from build123d import *

# Parameters (mm, degrees)
F2_SIZE = 1
F3_R    = 1


with BuildPart() as f1:
    # F0 (on Front) → F1 (revolve)
    with BuildSketch(Plane.XZ):
        Polygon((0, 4), (0, 0), (25, 0), (25, 4), (19.505045, 6), (14, 6), (14, 4), align=None)
    revolve(axis=Axis((10.323764, 0, 0), (1, 0, 0)))

    # F2
    f2_edges = [f1.edges().sort_by_distance(p)[0] for p in [
        (0, 0, -4),
    ]]
    chamfer(f2_edges, length=F2_SIZE)

    # F3
    f3_edges = [f1.edges().sort_by_distance(p)[0] for p in [
        (25, 0, -4),
    ]]
    fillet(f3_edges, radius=F3_R)


solid = f1.part
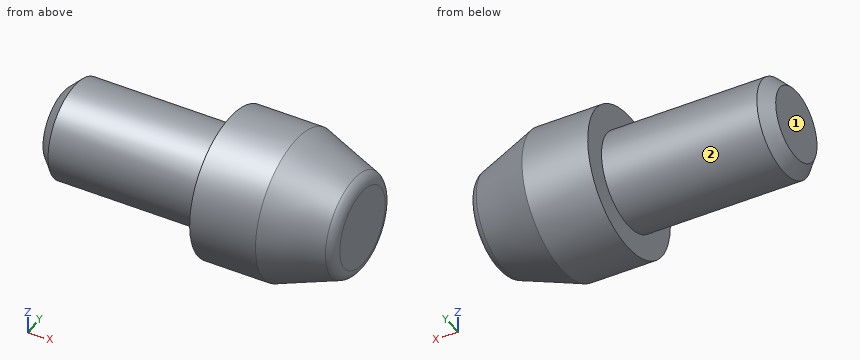
Part model, mm, in its own coordinate system. Face numbers are marked on the shaded views. A direction names the side the tool comes from. Coordinates: 2 decimals unless noted, no trailing zeros. Loops run counter-clockwise (first coordinate to the right, second up) from the corner with the lowest first, then second, coordinate; pieces in that order, holes last. Notation, with made-up numbers: (19, 65.25) -> (35, 65.25) arc R31 cw to (35, 103.25) -> close; hole circle Ø7 at (-31.75, 30.5). An arc over 180 degrees is marked (long way). Use a Markdown table: item, result. Add a question column.
Item 1: Band-saw the part on D-D on x = 11.5. Write the cut outline in (y, z), plus the area to 3 significant figures.
Item 2: Probe probe 1 along Z at (x, y) = (5, 0); probe 2 along Z at (x, y) = (12.5, -3.5); probe 3 along X at (y, z) = (4, 4). List the from-to ranges inside material, lowest first.
Item 3: Band-saw the part on A-A on y = 0. Write the cut outline in (x, z).
Item 4: Which spindle directions (+Z, -Z, +X, -X, +Y, -Y) get a long thin tool onto all of the face, cutting with end or side? Do the marked faces 1 and 2. Say none if no direction does.
Item 5: Flat gauge pins, fed straight in: P1, Ø4, axis at x = 14, z = -3, coming from the -Y side; P2, Ø2, axis at x = 10.5, y = 1, coming from the +Z side; P3, Ø1, axis at x = 15, y = -1.5, coming from the -Z side. Where does each tip first touch, or does it go through?
Item 6: Band-saw the part on C-C on x = 16.75. Write the cut outline in (y, z), plus the area to 3 significant figures.
Geometry says:
| question | item | result |
|---|---|---|
| 1 | outline | circle Ø8 at (0, 0) |
| 1 | area | 50.3 mm² |
| 2 | probe 1 | -4 to 4 |
| 2 | probe 2 | -1.94 to 1.94 |
| 2 | probe 3 | 14 to 20.45 |
| 3 | outline | (0, -3) -> (1, -4) -> (14, -4) -> (14, -6) -> (19.51, -6) -> (24.34, -4.24) arc R1 ccw to (25, -3.3) -> (25, 3.3) arc R1 ccw to (24.34, 4.24) -> (19.51, 6) -> (14, 6) -> (14, 4) -> (1, 4) -> (0, 3) -> close |
| 4 | face 1 | +Z, -Z, -X, +Y, -Y |
| 4 | face 2 | -X |
| 5 | P1 | y = -5.92 |
| 5 | P2 | z = 4 |
| 5 | P3 | z = -5.92 |
| 6 | outline | circle Ø12 at (0, 0) |
| 6 | area | 113 mm² |
